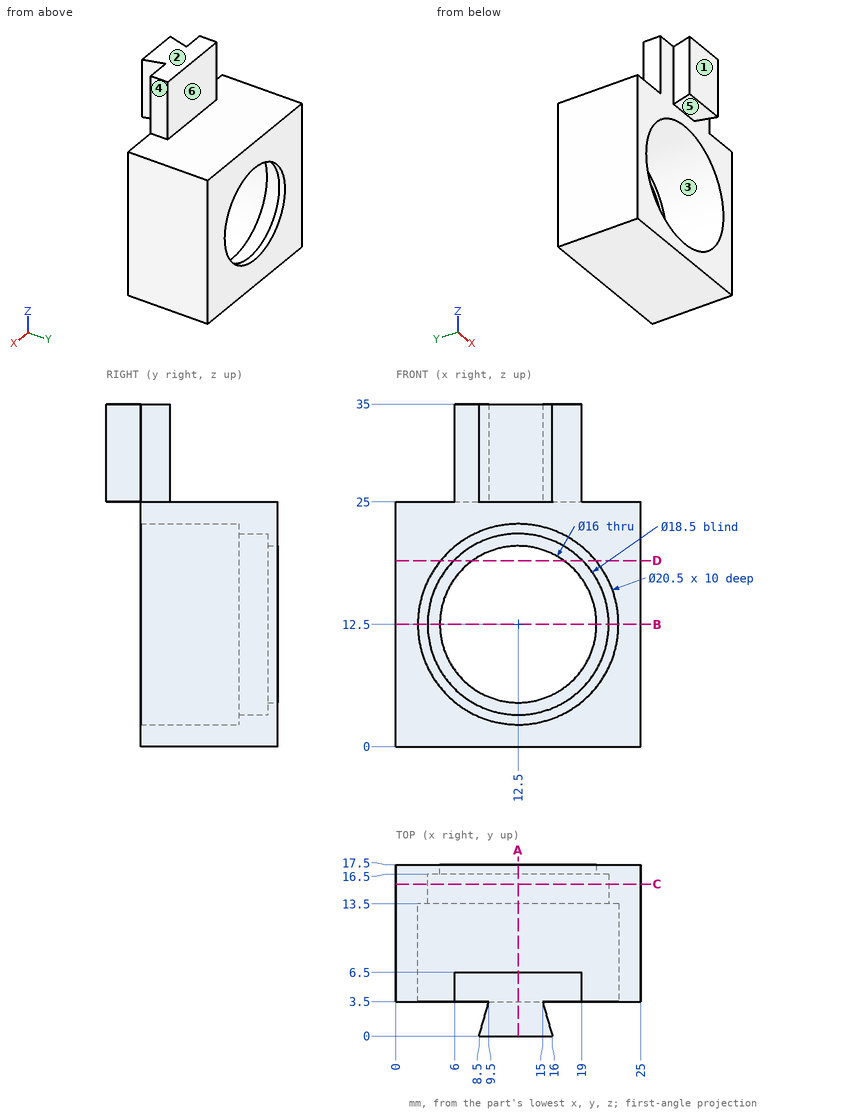
Here's the drawing with two shaded views (mm, measured from the low corner). I have some questions. A direction names the side the tool comes from. Give positions to 0.01 mm unless a question says otherwise; leave off trailing zeros. Loops run counter-clockwise (first coordinate to the right, second up) from the corner with the lowest first, then second, coordinate; pieces in that order, holes last. Notation, with made-up numbers: (73, 66) -> (102, 66) arc R15 cw to (102, 80) -> close; hole circle Ø4 at (-39, 10.25). An arc over 180 degrees is marked (long way). Use one line per item in the form item = value.
1) If we section it at B-B (z = 12.5): Please give me the cut outline in (x, y), plus the area to 3 significant figures.
Answers:
outline = (0, 3.5) -> (2.25, 3.5) -> (2.25, 13.5) -> (3.25, 13.5) -> (3.25, 16.5) -> (4.5, 16.5) -> (4.5, 17.5) -> (0, 17.5) -> close; (20.5, 16.5) -> (21.75, 16.5) -> (21.75, 13.5) -> (22.75, 13.5) -> (22.75, 3.5) -> (25, 3.5) -> (25, 17.5) -> (20.5, 17.5) -> close
area = 73.5 mm²
2) If we section it at D-D (z = 19): Please give me the cut outline in (x, y), plus the area to 3 significant figures.
Answers:
outline = (0, 3.5) -> (4.57, 3.5) -> (4.57, 13.5) -> (5.92, 13.5) -> (5.92, 16.5) -> (7.84, 16.5) -> (7.84, 17.5) -> (0, 17.5) -> close; (17.16, 16.5) -> (19.08, 16.5) -> (19.08, 13.5) -> (20.43, 13.5) -> (20.43, 3.5) -> (25, 3.5) -> (25, 17.5) -> (17.16, 17.5) -> close
area = 143 mm²
3) Will these pins go through, and if not, where does the flat tip stop? pin 1 (8 mm diameter, centred on x = 15.5, z = 29.5, fed in from +Y); pin 2 (7 mm diameter, centred on x = 15.5, y = 11, fed in from +Z); pin 3 (12.5 mm diameter, centred on x = 12.5, z = 12.5, fed in from +Y); pin 4 (6 mm diameter, centred on x = 10, z = 8, fed in from -Y).
Answers:
pin_1 = 6.5
pin_2 = 25
pin_3 = through
pin_4 = 16.5
4) I need wall thicknesses on line 1 along Z through (x, y) = (12.5, 14.35); line 2 along Z through (x, y) = (12.5, 17); line 3 along X through (y, z) = (7.25, 16.5). Which ranges of each line are inside material? Lowest first, please.
Answers:
line_1 = 0 to 3.25, 21.75 to 25
line_2 = 0 to 4.5, 20.5 to 25
line_3 = 0 to 3.06, 21.94 to 25
5) We'd pull the mould along Z, two halves only. Please class the marked faces 1, 2 and 3: released by +Z, released by -Z, zero draft, split by the parting line, or undercut.
Answers:
face_1 = zero draft
face_2 = released by +Z
face_3 = undercut
6) If we section it at A-A (x = 12.5): Please give me the cut outline in (y, z), plus the area to 4 significant figures.
Answers:
outline = (0, 25) -> (3.5, 25) -> (3.5, 22.75) -> (13.5, 22.75) -> (13.5, 21.75) -> (16.5, 21.75) -> (16.5, 20.5) -> (17.5, 20.5) -> (17.5, 25) -> (6.5, 25) -> (6.5, 35) -> (0, 35) -> close; (3.5, 0) -> (17.5, 0) -> (17.5, 4.5) -> (16.5, 4.5) -> (16.5, 3.25) -> (13.5, 3.25) -> (13.5, 2.25) -> (3.5, 2.25) -> close
area = 138.5 mm²
7) If we section it at C-C (y = 15.5): Please give me the cut outline in (x, z).
Answers:
outline = (0, 0) -> (25, 0) -> (25, 25) -> (0, 25) -> close; hole circle Ø18.5 at (12.5, 12.5)
8) For the marked faces 4, 5 and 6, which set-ups out of +Z, -Z, +X, -X, +Y, -Y let a thin tool reach every point of the face, with its end or its side?
Answers:
face_4 = +Z, +X, +Y, -Y
face_5 = -Z, +X, -X, -Y
face_6 = +Z, +X, -X, +Y
